Here's how the part is built. I have some questions about the finished solid (model axes, mm). A direction names the side the tool comes from. Round coordinates to 2 decimals unless told otherwise and drop trailing zeros. Order: outer loops, then holes, each group sorted by start corner. A loop starts at its lowest first (then second) coordinate and runs counter-clockwise, first axis right, second up.
```python
from build123d import *

# Parameters (mm, degrees)
F0_W     = 177.8
F0_H     = 127
F0_W_2   = 127
F0_H_2   = 76.2
F1_DEPTH = 127
F2_DEPTH = 101.6
F3_R     = 12.7
F4_R     = 12.7


with BuildPart() as f1:
    # F0 (on Top) → F1 (new body)
    with BuildSketch(Plane.XY):
        with Locations((7.560192, -20.097298)):
            Rectangle(F0_W, F0_H)
        with Locations((7.560192, -20.097298)):
            Rectangle(F0_W_2, F0_H_2, mode=Mode.SUBTRACT)
        with Locations((7.560192, -20.097298)):
            Rectangle(F0_W_2, F0_H_2)
    extrude(amount=F1_DEPTH)

    # F0 (on Top) → F2 (cut)
    with BuildSketch(Plane.XY):
        with Locations((7.560192, -20.097298)):
            Rectangle(F0_W_2, F0_H_2)
    extrude(amount=F2_DEPTH, mode=Mode.SUBTRACT)

    # F3
    f3_edges = [f1.edges().sort_by_distance(p)[0] for p in [
        (-55.939808, 18.002702, 50.8),
        (-55.939808, -58.197298, 50.8),
        (71.060192, 18.002702, 50.8),
        (71.060192, -58.197298, 50.8),
    ]]
    fillet(f3_edges, radius=F3_R)

    # F4
    f4_edges = [f1.edges().sort_by_distance(p)[0] for p in [
        (96.460192, -83.597298, 63.5),
        (96.460192, 43.402702, 63.5),
        (-81.339808, -83.597298, 63.5),
        (-81.339808, 43.402702, 63.5),
    ]]
    fillet(f4_edges, radius=F4_R)


solid = f1.part
```
1) I'm going to push a flat-ended pin straight in: pin 1 (6 mm diameter, centred on x = 5, y = -15, fed in from -Z). Where does the tip first touch, or does it pass through?
2) We'd pull the mould along Y, two halves only. Please class faces 1 (the cylindrical face through (92.64, 39.78, 64.39)), 2 (the flat face through (6, -83.597, 63)), 3 (the cylindrical face through (-52.1, 14.4, 51.5)), 4 (the flat face through (6, 23, 0)): +Y half, -Y half, draft (parallel to the pull), parting line (faces both ways), or undercut.
3) I need wall thicknesses on line 1 (Y direction, x = -41, z = 20); line 2 (X direction, y = -28, z = 24); line 3 (Z direction, x = -36.5, y = 6). Which ranges of each line are inside material? Lowest first, please.
4) If we section it at A-A (z = 85): Write out the boundary of the cut face in (x, y), plus the area to 3 significant figures.
5) If we section it at B-B (x = -27): Write out the boundary of the cut face in (y, z), plus the area to 3 significant figures.
6) For faces 5 (the flat face through (7, -58.197, 50)), 6 (the cylindrical face through (-77.7, 39.6, 64.4)), which set-ups out of +Z, -Z, +X, -X, +Y, -Y let a thin tool reach every point of the face, with its end or its side?
7) If we section it at C-C (y = -31.5): Write out the boundary of the cut face in (x, z).
Solutions:
1. pin 1: stops at z = 101.6
2. face 1: +Y half
2. face 2: -Y half
2. face 3: undercut
2. face 4: draft
3. line 1: y = -83.6 to -58.2, 18 to 43.4
3. line 2: x = -81.34 to -55.94, 71.06 to 96.46
3. line 3: z = 101.6 to 127
4. outline: (-81.34, -70.9) arc R12.7 ccw to (-68.64, -83.6) - (83.76, -83.6) arc R12.7 ccw to (96.46, -70.9) - (96.46, 30.7) arc R12.7 ccw to (83.76, 43.4) - (-68.64, 43.4) arc R12.7 ccw to (-81.34, 30.7) - close; hole (-55.94, -45.5) arc R12.7 ccw to (-43.24, -58.2) - (58.36, -58.2) arc R12.7 ccw to (71.06, -45.5) - (71.06, 5.3) arc R12.7 ccw to (58.36, 18) - (-43.24, 18) arc R12.7 ccw to (-55.94, 5.3) - close
4. area: 12,900 mm2
5. outline: (-83.6, 0) - (-58.2, 0) - (-58.2, 101.6) - (18, 101.6) - (18, 0) - (43.4, 0) - (43.4, 127) - (-83.6, 127) - close
5. area: 8,390 mm2
6. face 5: -Z
6. face 6: +Z, -Z, -X, +Y
7. outline: (-81.34, 0) - (-55.94, 0) - (-55.94, 101.6) - (71.06, 101.6) - (71.06, 0) - (96.46, 0) - (96.46, 127) - (-81.34, 127) - close
